Build history of the part. All positions in model axes, mm. A direction names the side the tool comes from. Round coordinates to 2 decimals unless told otherwise and drop trailing zeros. Write each loop counter-clockwise with the first axis right and the second up, starting at its lowest first coordinate (ties: lowest second). Pieces come first, ordered by that corner, then holes. Notation, with made-up numbers: (-17.5, -13.75) - (21.5, -13.75) arc R13 ccw to (21.5, 8.25) - close; hole circle Ø11 at (20.5, -22.75). An arc over 180 degrees is marked (long way). Write each question's results on one line, items separated by ' | '.
from build123d import *

# Parameters (mm, degrees)
BOSS_EXTRUDE1_DEPTH = 25
SHELL13_T           = -3
SKETCH3_R           = 3
CUT_EXTRUDE2_DEPTH  = 3
SKETCH4_W           = 10
SKETCH4_H           = 1
SKETCH4_W_2         = 1
SKETCH4_H_2         = 10
SKETCH4_W_3         = 7
BOSS_EXTRUDE2_DEPTH = 5
SKETCH5_R           = 3
CUT_EXTRUDE3_DEPTH  = 30


with BuildPart() as part:
    # Sketch1 → Boss-Extrude1 (new body)
    with BuildSketch(Plane.XY):
        with BuildLine():
            Line((15, -15), (15, 15))
            Line((15, 15), (-15, 15))
            Line((-15, 15), (-15, -15))
            ThreePointArc((-15, -15), (0, -18.870680067), (15, -15))
        make_face()
    extrude(amount=BOSS_EXTRUDE1_DEPTH)

    # Shell13
    shell13_openings = [part.faces().sort_by_distance(p)[0] for p in [
        (0, -1.327259688, 0),
    ]]
    offset(amount=SHELL13_T, openings=shell13_openings, kind=Kind.INTERSECTION)

    # Sketch3 → Cut-Extrude2 (cut)
    with BuildSketch(Plane(origin=(0, 0, 22), x_dir=(-1, 0, 0), z_dir=(0, 0, -1))):
        with Locations((0.010259738, 0.007572697)):
            Circle(SKETCH3_R)
    extrude(amount=-CUT_EXTRUDE2_DEPTH, mode=Mode.SUBTRACT)

    # Sketch4 → Boss-Extrude2 (add)
    with BuildSketch(Plane(origin=(0, 0, 0), x_dir=(-1, 0, 0), z_dir=(0, 0, -1))):
        with Locations((0, 13.5)):
            Rectangle(SKETCH4_W, SKETCH4_H)
        with Locations((-13.5, 0)):
            Rectangle(SKETCH4_W_2, SKETCH4_H_2)
        with Locations((0, -17.5)):
            Rectangle(SKETCH4_W_3, SKETCH4_H)
        with Locations((13.5, 0)):
            Rectangle(SKETCH4_W_2, SKETCH4_H_2)
    extrude(amount=BOSS_EXTRUDE2_DEPTH)

    # Sketch5 → Cut-Extrude3 (cut)
    with BuildSketch(Plane(origin=(15, 0, 0), x_dir=(0, 0, -1), z_dir=(1, 0, 0))):
        with Locations(Location((-15, 0, 0), (0, 0, 90))):
            Circle(SKETCH5_R)
    extrude(amount=-CUT_EXTRUDE3_DEPTH, mode=Mode.SUBTRACT)


solid = part.part
(1) Slice it at D-D, the plane z = 20.5. Write the cut outline in (x, y).
Worked answers:
outline: (-15, -15) arc R31 ccw to (15, -15) - (15, 15) - (-15, 15) - close; hole (-12, -13.17) arc R28 ccw to (12, -13.17) - (12, 12) - (-12, 12) - close
(2) Slice it at B-B, the plane z = 15. Write the cut outline in (x, y).
Worked answers:
outline: (-15, -15) arc R31 ccw to (15, -15) - (15, -3) - (12, -3) - (12, -13.17) arc R28 cw to (-12, -13.17) - (-12, -3) - (-15, -3) - close; (-15, 3) - (-12, 3) - (-12, 12) - (12, 12) - (12, 3) - (15, 3) - (15, 15) - (-15, 15) - close
(3) Two-plate mould, pull along X, no slides. Class faces 1 (the flat face through (-3, -2, 22)), 2 (the flat face through (0, -18, -2)), 3 (the flat face through (15, 0, 10)): released by +X, released by -X, zero draft, split by the parting line, or undercut.
Worked answers:
face 1: undercut | face 2: zero draft | face 3: released by +X
(4) Tool access for faces 4 (the flat face through (0, 14, -2)), 5 (the flat face through (-5, 13.5, -2.5)), 6 (the flat face through (-12, 0, 11)): list every direction of +Z, -Z, +X, -X, +Y, -Y with a clear straight run to the whole face (end or side of a thin tool).
Worked answers:
face 4: -Z, +X, -X, +Y | face 5: -Z, -X, +Y, -Y | face 6: -Z
(5) Slice it at A-A, the plane z = -1.5. Write the cut outline in (x, y), and give its area (3 significant figures).
Worked answers:
outline: (-14, -5) - (-13, -5) - (-13, 5) - (-14, 5) - close; (-5, 13) - (5, 13) - (5, 14) - (-5, 14) - close; (-3.5, -18) - (3.5, -18) - (3.5, -17) - (-3.5, -17) - close; (13, -5) - (14, -5) - (14, 5) - (13, 5) - close | area: 37.0 mm2
(6) Flat gauge pins, fed straight in: pin 1 Ø2.5 at (x, z) = (-0.5, -2.5) entering from -Y; pin 2 Ø0.8 at (x, z) = (13.5, -2.5) entering from +Y; pin 3 Ø1.5 at (x, z) = (6, -2) entering from +Y; pin 4 Ø0.8 at (x, z) = (-13.5, -2) entering from -Y. Where does each tip first touch, or does it go through?
Worked answers:
pin 1: stops at y = -18 | pin 2: stops at y = 5 | pin 3: passes through | pin 4: stops at y = -5
(7) Drill centre lines: probe 1 along X at (y, z) = (2, 17.75); probe 2 along Z at (x, y) = (14.35, 0); probe 3 along X at (y, z) = (2, -3.25). Where is each one in solid material? Low to high. Write a range as [from, to].
Worked answers:
probe 1: x = [-15, -12], [12, 15] | probe 2: z = [0, 12], [18, 25] | probe 3: x = [-14, -13], [13, 14]
(8) Slice it at C-C, the plane y = -9. Write the cut outline in (x, z), and give its area (3 significant figures).
Worked answers:
outline: (-15, 0) - (-12, 0) - (-12, 22) - (12, 22) - (12, 0) - (15, 0) - (15, 25) - (-15, 25) - close | area: 222 mm2
